The figure shows three views and two pictorial views of one solid part (mm, origin at its lowest corner). Answer the questions. Coordinates: 2 decimals unless noted, no trailing zeros. Loops run counter-clockwise (first coordinate to the right, second up) from the corner with the lowest first, then second, coordinate; pieces in that order, holes last. Notation, with made-up numbers: M -34.75,71 L -21.75,71 A27 cw -21.75,94 Z; hole C 18,-31.75 d9. An arc over 180 degrees is marked long. Return JSON: item names as keys, results as strings. Group by question number.
1. Section B-B (x = 22) is taken. Write down the section's boundary in (y, z), then the cut area to 3 significant figures.
2. Straight lines are drawn through the part: L1, parallel to Y at x = 26.5, z = 12.5; L2, parallel to Y at x = 50, z = 4; L3, parallel to Z at x = 43, y = 6.75. For each, find the intervals that lie inside material, in ascending order. Write a range as from..to.
3. Section A-A (z = 9.5) is taken. Write down the section's boundary in (x, y), then the cut area to 3 significant figures.
4. Section C-C (y = 24) is taken. Write down the section's boundary in (x, z), then the cut area to 3 significant figures.
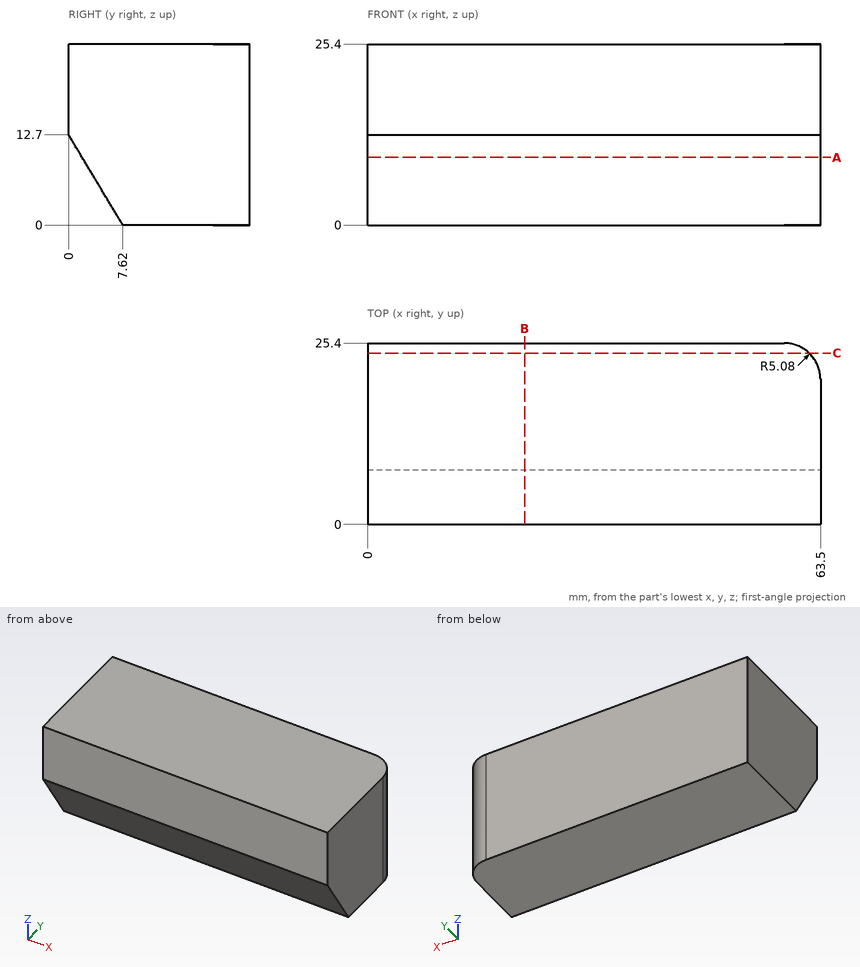
Worked out:
{
 "1": {"outline": "M 0,12.7 L 7.62,0 L 25.4,0 L 25.4,25.4 L 0,25.4 Z", "area": "597 mm^2"},
 "2": {"L1": "0.12..25.4", "L2": "5.22..25.4", "L3": "1.45..25.4"},
 "3": {"outline": "M 0,1.92 L 63.5,1.92 L 63.5,20.32 A5.08 ccw 58.42,25.4 L 0,25.4 Z", "area": "1,490 mm^2"},
 "4": {"outline": "M 0,0 L 61.92,0 L 61.92,25.4 L 0,25.4 Z", "area": "1,570 mm^2"}
}
